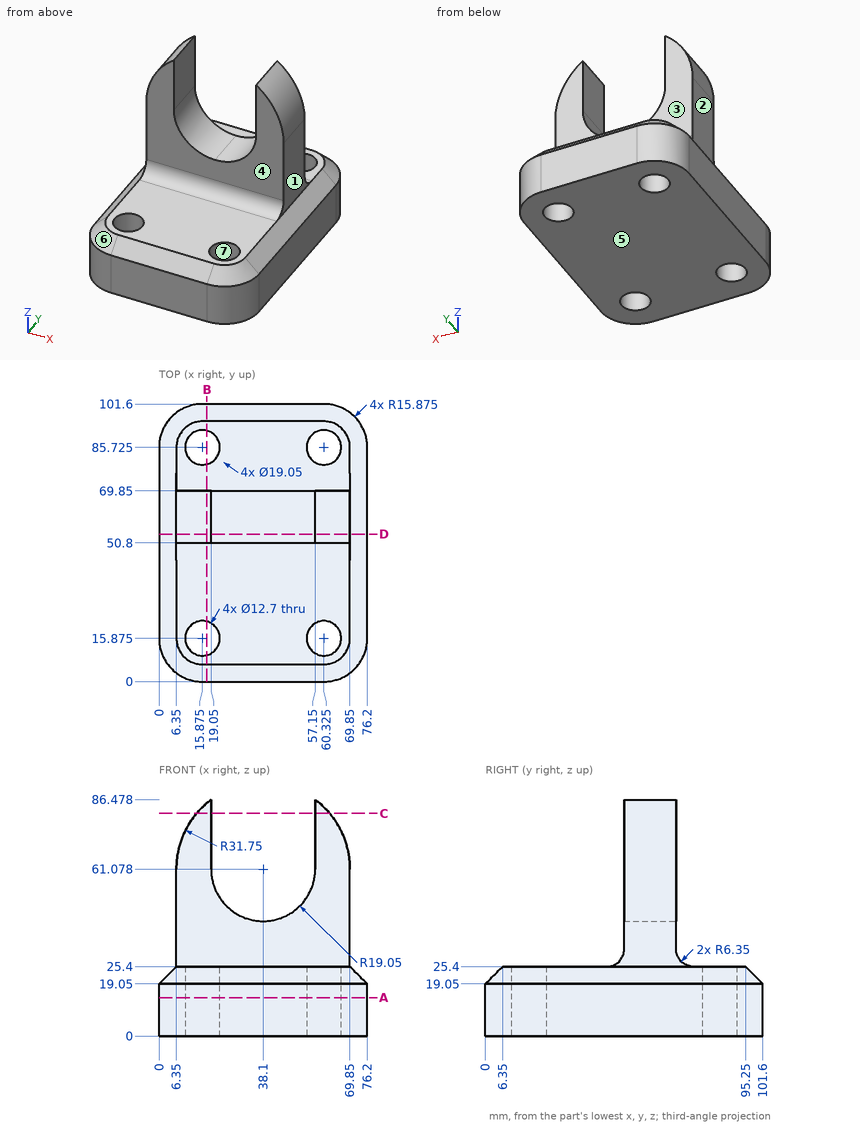
Here's the drawing with two shaded views (mm, measured from the low corner). I have some questions. A direction names the side the tool comes from. Round coordinates to 2 decimals unless told otherwise and drop trailing zeros. Order: outer loops, then holes, each group sorted by start corner. A loop starts at its lowest first (then second) coordinate and runs counter-clockwise, first axis right, second up. Notation, with made-up numbers: (-16.5, -21) -> (-7.5, -21) arc R22 cw to (-7.5, -3) -> close; hole circle Ø11 at (-8.5, 70.5). An arc over 180 degrees is marked (long way). Use a Markdown table: item, result. Add a question column.
(1) For the marked faces 1, 2, 3 and 4, which set-ups out of +Z, -Z, +X, -X, +Y, -Y let a thin tool reach every point of the face, with its end or its side?
(2) Suppose I cut it at B-B, the plane x = 17.5. Please give me the cut outline in (y, z), and give its area (3 significant figures).
(3) If we mould it in two halves opening along X, with no side actions, what happens to the marked faces 5, 6 and 7? For each: released by +X, released by -X, zero draft, split by the parting line, or undercut.
(4) For pin 1 Ø14.5 at (x, y) = (15.875, 85.725) entering from +Z; pin 2 Ø10 at (x, y) = (60.325, 15.875) entering from -Z; pin 3 Ø21 at (y, z) = (60.5, 69.5) entering from -X; pin 4 Ø12 at (x, y) = (10.5, 54) entering from +Z, each with a flat end and sliding along its axis, tell me the tip position at first contact or that it passes through.
(5) Suppose I cut it at C-C, the plane z = 81.5. Please give me the cut outline in (x, y).
(6) Suppose I cut it at A-A, the plane z = 14. Count the separate pieces of the cut face and the enclosed holes in it, and give its area (3 significant figures).
(7) Suppose I cut it at D-D, the plane y = 54. Please give me the cut outline in (x, z), and give its area (3 significant figures).
(8) I need wall thicknesses on line 1 along X through (y, z) = (83, 19); line 2 along Y through (x, z) = (62.5, 70); line 3 along X through (y, z) = (88.5, 13.5) (1 decimal). Which ranges of each line are inside material? Lowest first, please.
Verdict:
| question | item | result |
|---|---|---|
| 1 | face 1 | +Z, +X, +Y, -Y |
| 1 | face 2 | +Z, -X, +Y, -Y |
| 1 | face 3 | +Z, +X, -X, +Y |
| 1 | face 4 | +Z, +X, -X, -Y |
| 2 | outline | (0, 0) -> (9.74, 0) -> (9.74, 25.4) -> (6.35, 25.4) -> (0, 19.05) -> close; (22.01, 0) -> (79.59, 0) -> (79.59, 25.4) -> (76.2, 25.4) arc R6.35 cw to (69.85, 31.75) -> (69.85, 85.24) -> (50.8, 85.24) -> (50.8, 31.75) arc R6.35 cw to (44.45, 25.4) -> (22.01, 25.4) -> close; (91.86, 0) -> (101.6, 0) -> (101.6, 19.05) -> (95.25, 25.4) -> (91.86, 25.4) -> close |
| 2 | area | 3,070 mm2 |
| 3 | face 5 | zero draft |
| 3 | face 6 | released by -X |
| 3 | face 7 | undercut |
| 4 | pin 1 | z = 25.4 |
| 4 | pin 2 | through |
| 4 | pin 3 | x = 6.35 |
| 4 | pin 4 | z = 84.35 |
| 5 | outline | (13.79, 50.8) -> (19.05, 50.8) -> (19.05, 69.85) -> (13.79, 69.85) -> close; (57.15, 50.8) -> (62.41, 50.8) -> (62.41, 69.85) -> (57.15, 69.85) -> close |
| 6 | separate pieces | 1 |
| 6 | enclosed holes | 4 |
| 6 | area | 7,020 mm2 |
| 7 | outline | (0, 0) -> (76.2, 0) -> (76.2, 19.05) -> (69.85, 25.4) -> (69.85, 61.08) arc R31.75 ccw to (57.15, 86.48) -> (57.15, 61.08) arc R19.05 cw to (19.05, 61.08) -> (19.05, 86.48) arc R31.75 ccw to (6.35, 61.08) -> (6.35, 25.4) -> (0, 19.05) -> close |
| 7 | area | 4,040 mm2 |
| 8 | line 1 | 0 to 10.14, 21.61 to 54.59, 66.06 to 76.2 |
| 8 | line 2 | 50.8 to 69.85 |
| 8 | line 3 | 0.2 to 10.2, 21.6 to 54.6, 66 to 76 |
